Answer from the drawing. Dimensions are ordinates in mm from the lowest x, y and z of the part. A direction names the side the tool comes from. Coordinates: 2 decimals unless noted, no trailing zeros. Write each loop counter-clockwise with the first axis right and the second up, starting at its lowest first coordinate (ties: lowest second). Pieces come first, ordered by that corner, then holes.
1) The part is cut by section B-B (z = 5.5). Give the number of separate pieces and of enclosed holes in the cut face, then the cut area to 3 significant figures.
2) The part is cut by section D-D (y = 5.6). Determine the outline of the cut face in (x, z) (1 decimal).
3) Which of the six approach directions +Z, -Z, +X, -X, +Y, -Y give full straight-line access (tool end or side, diameter ignored) to the marked faces 1, 2 and 3?
4) Each of these flat-tipped pins is pushed along its axis until it touches: pin 1 Ø3.5 at (x, z) = (20, 8) entering from +Y; pin 2 Ø3.5 at (x, z) = (31, 14) entering from +Y. Where does it stop, or does it pass through?
5) Find the intervals of material crossed by line 1 (X direction, y = 2.85, z = 5.5); line 2 (X direction, y = 5.35, z = 19) (1 decimal); line 3 (Y direction, x = 6.5, z = 29), in increasing order.
6) The part is cut by section A-A (x = 30). Determine the outline of the cut face in (y, z).
7) Determine the mould class of the marked faces 4, 5 and 6 for opening direction Z: +Z half, -Z half, draft (parallel to the pull), parting line (faces both ways), or undercut.
8) The part is cut by section C-C (y = 1.15). Determine the outline of the cut face in (x, z).
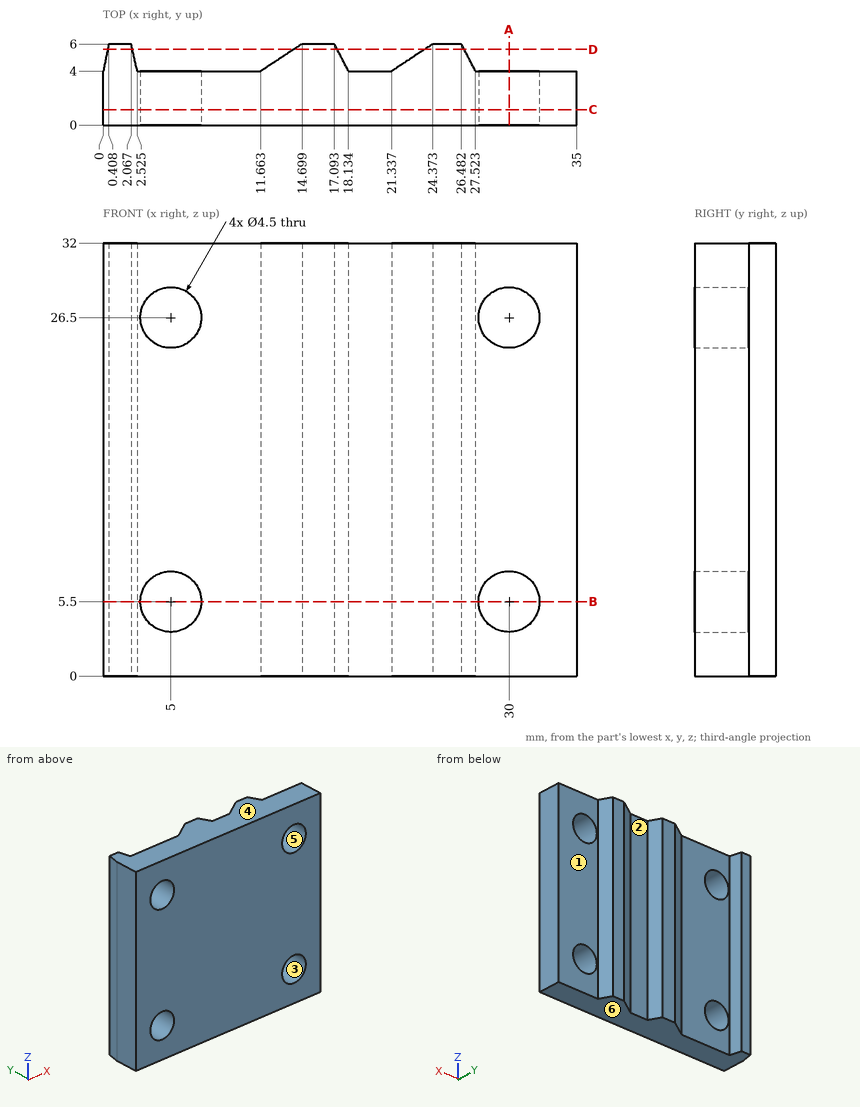
Reported:
1. separate pieces: 3
1. enclosed holes: 0
1. area: 125 mm2
2. outline: (0.3, 0) - (2.2, 0) - (2.2, 32) - (0.3, 32) - close; (14.1, 0) - (17.3, 0) - (17.3, 32) - (14.1, 32) - close; (23.8, 0) - (26.7, 0) - (26.7, 32) - (23.8, 32) - close
3. face 1: +Z, -Z, +X, +Y
3. face 2: +Z, -Z, +Y
3. face 3: +Y, -Y
4. pin 1: stops at y = 4.27
4. pin 2: stops at y = 4
5. line 1: x = 0 to 2.75, 7.25 to 27.75, 32.25 to 35
5. line 2: x = 0.3 to 2.2, 13.7 to 17.4, 23.4 to 26.8
5. line 3: y = 0 to 4
6. outline: (0, 0) - (4, 0) - (4, 3.25) - (0, 3.25) - close; (0, 7.75) - (4, 7.75) - (4, 24.25) - (0, 24.25) - close; (0, 28.75) - (4, 28.75) - (4, 32) - (0, 32) - close
7. face 4: +Z half
7. face 5: undercut
7. face 6: -Z half
8. outline: (0, 0) - (35, 0) - (35, 32) - (0, 32) - close; hole circle Ø4.5 at (5, 5.5); hole circle Ø4.5 at (5, 26.5); hole circle Ø4.5 at (30, 5.5); hole circle Ø4.5 at (30, 26.5)
